Can you work these out from the model? Positions are in its coordinate system, mm. A direction names the side the tool comes from. Give positions to 0.01 mm unless a question says otherwise; leave off trailing zeros. Write each loop counter-clockwise with the first axis right and the second up, starting at its lowest first coordinate (ties: lowest second). Pieces come first, ordered by that corner, then holes. Notation, with made-up numbers: (71.25, 24.5) -> (93.25, 24.5) arc R21 ccw to (93.25, 52.5) -> close; hole circle Ø1 at (30.5, -11). An arc over 180 degrees is marked (long way). Answer as CSV lines item,"result". Start each with the question number.
1. If we mould it in two halves opening along Y, with no side actions, what happens to faces 5 (the face through (-197.39, -11.53, 30.03)), 6 (the face through (-231.29, 35.27, 30.53)), 7 (the face through (-241.7, 6.3, 28)), 8 (the face through (-207, 24.5, 31))? For each: pulls with the +Y half, pulls with the -Y half, needs draft (parallel to the pull), parting line crosses it, or undercut.
2. If we section it at A-A on x = -199: Write out the boundary of the cut face in (y, z), plus the area to 3 significant figures.
3. If we section it at C-C on y = -9: Write out the boundary of the cut face in (x, z).
4. I'm going to push flat-ended pins straight in: P1, Ø13.5, axis at x = -218.5, y = 0, coming from the -Z side; P2, Ø3, axis at x = -219.5, z = 30, coming from the -Y side; P3, Ø3, axis at y = 20.5, z = 30, coming from the +X side; P4, Ø1.2, axis at x = -187, y = -27.5, coming from the -Z side. Where does each tip first touch, or does it pass through?
5. On a 3-axis mill with a long thin cutter (end or side, diameter ignored), from which of +Z, -Z, +X, -X, +Y, -Y can I reach the whole of each face in a straight line? I mean faces 1 (the face through (-200.5, -9.07, 30.03)), 2 (the face through (-180.78, 18.15, 32.51)), 3 (the face through (-242, 24.5, 31)), 4 (the face through (-208, -24.5, 31)). Say none if no direction works.
6. I need wall thicknesses on line 1 (Y direction, x = -231, z = 30.6); line 2 (Y direction, x = -243, z = 30.75); line 3 (Y direction, x = -239.5, z = 31.3). Which ranges of each line are inside material? Lowest first, please. Write a range as [from, to].
```python
from build123d import *

# Parameters (mm, degrees)
SKETCH123_W             = 60
SKETCH123_H             = 45
PAD050_DEPTH            = 5
PAD099_DEPTH            = 1
SKETCH128_R             = 3
SKETCH128_R_2           = 1.5
PAD100_DEPTH            = 5
SKETCH223_R             = 2.25
POCKET090_DEPTH         = 5
BODY015_PLACEMENT_ANGLE = 180


with BuildPart() as part:
    # Sketch123 → Pad050 (new body)
    with BuildSketch(Plane.XY):
        with BuildLine():
            Line((-32, 24.5), (-20, 24.5))
            Line((-20, 24.5), (-20, 37.5))
            ThreePointArc((-10, 37.5), (-15, 42.5), (-20, 37.5))
            Line((-10, 24.5), (-10, 37.5))
            Line((-10, 24.5), (27.428932, 24.5))
            Line((27.428932, 24.5), (31.464466, 28.535534))
            ThreePointArc((38.535534, 21.464466), (38.535534, 28.535534), (31.464466, 28.535534))
            Line((32, 14.928932), (38.535534, 21.464466))
            Line((32, 14.928932), (32, -14.928932))
            Line((32, -14.928932), (38.535534, -21.464466))
            ThreePointArc((31.464466, -28.535534), (38.535534, -28.535534), (38.535534, -21.464466))
            Line((27.428932, -24.5), (31.464466, -28.535534))
            Line((27.428932, -24.5), (-10, -24.5))
            Line((-10, -24.5), (-10, -37.5))
            ThreePointArc((-20, -37.5), (-15, -42.5), (-10, -37.5))
            Line((-20, -24.5), (-20, -37.5))
            Line((-20, -24.5), (-32, -24.5))
            Line((-32, -24.5), (-32, 24.5))
        make_face()
        Rectangle(SKETCH123_W, SKETCH123_H, mode=Mode.SUBTRACT)
    extrude(amount=PAD050_DEPTH)

    # Sketch222 → Pad099 (join)
    with BuildSketch(Plane.XY):
        with BuildLine():
            Line((-31, 23.5), (-20, 23.5))
            Line((-20, 23.5), (-20, 37.5))
            ThreePointArc((-10, 37.5), (-15, 42.5), (-20, 37.5))
            Line((-10, 23.5), (-10, 37.5))
            Line((-10, 23.5), (26.426435, 23.5))
            Line((26.426435, 23.5), (31.465342, 28.53641))
            ThreePointArc((38.534658, 21.46359), (38.53641, 28.534658), (31.465342, 28.53641))
            Line((31, 13.932666), (38.534658, 21.46359))
            Line((31, 13.932666), (31, -13.927334))
            Line((31, -13.927334), (38.535909, -21.464841))
            ThreePointArc((31.464091, -28.535159), (38.535159, -28.535909), (38.535909, -21.464841))
            Line((26.43, -23.5), (31.464091, -28.535159))
            Line((26.43, -23.5), (-10, -23.5))
            Line((-10, -23.5), (-10, -37.5))
            ThreePointArc((-20, -37.5), (-15, -42.5), (-10, -37.5))
            Line((-20, -23.5), (-20, -37.5))
            Line((-20, -23.5), (-31, -23.5))
            Line((-31, -23.5), (-31, 23.5))
        make_face()
    extrude(amount=PAD099_DEPTH)

    # Sketch128 → Pad100 (join)
    with BuildSketch(Plane.XY):
        with Locations((-27, -5)):
            Circle(SKETCH128_R)
        with Locations((-27, -5)):
            Circle(SKETCH128_R_2, mode=Mode.SUBTRACT)
        with Locations((-27, -19)):
            Circle(SKETCH128_R)
        with Locations((-27, -19)):
            Circle(SKETCH128_R_2, mode=Mode.SUBTRACT)
        with Locations((17, 9)):
            Circle(SKETCH128_R)
        with Locations((17, 9)):
            Circle(SKETCH128_R_2, mode=Mode.SUBTRACT)
        with Locations((17, -19)):
            Circle(SKETCH128_R)
        with Locations((17, -19)):
            Circle(SKETCH128_R_2, mode=Mode.SUBTRACT)
    extrude(amount=PAD100_DEPTH)

    # Sketch223 → Pocket090 (cut)
    with BuildSketch(Plane.XY):
        with Locations((35, -25)):
            Circle(SKETCH223_R)
        with Locations((35, 25)):
            Circle(SKETCH223_R)
        with Locations((-15, 37.5)):
            Circle(SKETCH223_R)
        with Locations((-15, -37.5)):
            Circle(SKETCH223_R)
    extrude(amount=POCKET090_DEPTH, mode=Mode.SUBTRACT)


with BuildPart() as part_1:
    # Body015 placement: moved
    add(part.part.moved(Location((-216, 0, 33))).rotate(Axis((-216, 0, 33), (1, 0, 0)), BODY015_PLACEMENT_ANGLE))


solid = part_1.part
```
Computed values:
1,face 5,"undercut"
1,face 6,"undercut"
1,face 7,"needs draft"
1,face 8,"pulls with the +Y half"
2,outline,"(-24.5, 28) -> (-22.5, 28) -> (-22.5, 32) -> (-12, 32) -> (-12, 28) -> (-10.5, 28) -> (-10.5, 32) -> (-7.5, 32) -> (-7.5, 28) -> (-6, 28) -> (-6, 32) -> (16, 32) -> (16, 28) -> (17.5, 28) -> (17.5, 32) -> (20.5, 32) -> (20.5, 28) -> (22, 28) -> (22, 32) -> (22.5, 32) -> (22.5, 28) -> (24.5, 28) -> (24.5, 33) -> (-24.5, 33) -> close"
2,area,"89.0 mm2"
3,outline,"(-248, 28) -> (-246, 28) -> (-246, 32) -> (-202, 32) -> (-202, 28) -> (-200.5, 28) -> (-200.5, 32) -> (-197.5, 32) -> (-197.5, 28) -> (-196, 28) -> (-196, 32) -> (-186, 32) -> (-186, 28) -> (-184, 28) -> (-184, 33) -> (-248, 33) -> close"
4,P1,"stops at z = 32"
4,P2,"stops at y = -24.5"
4,P3,"stops at x = -177"
4,P4,"passes through"
5,face 1,"-Z"
5,face 2,"+Z, -Z, +X"
5,face 3,"+Z, -Z, -X, +Y"
5,face 4,"+Z, -Z, -Y"
6,line 1,"y = [-42.5, -39.75], [-35.25, -22.5], [22.5, 35.25], [39.75, 42.5]"
6,line 2,"y = [-24.5, -22.5], [2, 3.5], [6.5, 8], [16, 17.5], [20.5, 22], [22.5, 24.5]"
6,line 3,"y = [-24.5, -22.5], [22.5, 24.5]"
